from build123d import *

# Parameters (mm, degrees)
MODEL_W                 = 3
MODEL_H                 = 3
SALIENTE_EXTRUIR1_DEPTH = 3


with BuildPart() as part:
    # Model → Saliente-Extruir1 (new body)
    with BuildSketch(Plane.XY):
        with BuildLine():
            Line((12.639309496, 299.028131514), (48.639309496, 299.028131514))
            ThreePointArc((48.639309496, 299.028131514), (51.821290011, 297.71011203), (53.139309496, 294.528131514))
            Line((53.139309496, 294.528131514), (53.139309496, 276.528131514))
            ThreePointArc((53.139309496, 276.528131514), (51.821290011, 273.346150999), (48.639309496, 272.028131514))
            Line((48.639309496, 272.028131514), (12.639309496, 272.028131514))
            ThreePointArc((12.639309496, 272.028131514), (9.457328981, 273.346150999), (8.139309496, 276.528131514))
            Line((8.139309496, 276.528131514), (8.139309496, 294.528131514))
            ThreePointArc((8.139309496, 294.528131514), (9.457328981, 297.71011203), (12.639309496, 299.028131514))
        make_face()
        with Locations((12.639309496, 294.528131514)):
            Rectangle(MODEL_W, MODEL_H, mode=Mode.SUBTRACT)
        with Locations((21.639309496, 294.528131514)):
            Rectangle(MODEL_W, MODEL_H, mode=Mode.SUBTRACT)
        with Locations((30.639309496, 294.528131514)):
            Rectangle(MODEL_W, MODEL_H, mode=Mode.SUBTRACT)
        with Locations((39.639309496, 294.528131514)):
            Rectangle(MODEL_W, MODEL_H, mode=Mode.SUBTRACT)
        with Locations((48.639309496, 294.528131514)):
            Rectangle(MODEL_W, MODEL_H, mode=Mode.SUBTRACT)
        with Locations((12.639309496, 276.528131514)):
            Rectangle(MODEL_W, MODEL_H, mode=Mode.SUBTRACT)
        with Locations((21.639309496, 276.528131514)):
            Rectangle(MODEL_W, MODEL_H, mode=Mode.SUBTRACT)
        with Locations((30.639309496, 276.528131514)):
            Rectangle(MODEL_W, MODEL_H, mode=Mode.SUBTRACT)
        with Locations((39.639309496, 276.528131514)):
            Rectangle(MODEL_W, MODEL_H, mode=Mode.SUBTRACT)
        with Locations((48.639309496, 276.528131514)):
            Rectangle(MODEL_W, MODEL_H, mode=Mode.SUBTRACT)
        with Locations((12.639309496, 285.528131514)):
            Rectangle(MODEL_W, MODEL_H, mode=Mode.SUBTRACT)
        with Locations((21.639309496, 285.528131514)):
            Rectangle(MODEL_W, MODEL_H, mode=Mode.SUBTRACT)
        with Locations((30.639309496, 285.528131514)):
            Rectangle(MODEL_W, MODEL_H, mode=Mode.SUBTRACT)
        with Locations((39.639309496, 285.528131514)):
            Rectangle(MODEL_W, MODEL_H, mode=Mode.SUBTRACT)
        with Locations((48.639309496, 285.528131514)):
            Rectangle(MODEL_W, MODEL_H, mode=Mode.SUBTRACT)
    extrude(amount=SALIENTE_EXTRUIR1_DEPTH)


solid = part.part
Work out the finished part from the listing and answer in its coordinate system (mm). Coordinates: 2 decimals unless noted, no trailing zeros. Order: outer loops, then holes, each group sorted by start corner. A loop starts at its lowest first (then second) coordinate and runs counter-clockwise, first axis right, second up. Notation, with made-up numbers: (61.5, 4.25) - (107.5, 4.25) arc R9 ccw to (107.5, 16.25) - close; hole circle Ø1 at (14, 3.5). An arc over 180 degrees is marked (long way). Put each result on its own line as item: value. Start each with the question number.
1) Find section B-B (z = 2.2). State how many separate pieces and enclosed holes the cut face has, plus the area to 3 significant figures.
2) Find the intervals of material crossed by line 1 (X direction, y = 294, z = 0.45); line 2 (Y direction, x = 30, z = 2.95); line 3 (X direction, y = 295, z = 2.5), in increasing order. Write a range as from..to.
3) Find section A-A (y = 285.75). Give the vertices of the cut face in (x, z).
4) Find section C-C (y = 275.5). Give the vertices of the cut face in (x, z), plus the area to 3 significant figures.
5) For a pull along X with two mould halves and no side action, classify faces 1 (the flat face through (40, 278.028, 1)), 2 (the cylindrical face through (51.79, 297.74, 1.48)) as released by +X, released by -X, zero draft, split by the parting line, or undercut.
Results list:
1. separate pieces: 1
1. enclosed holes: 15
1. area: 1,060 mm^2
2. line 1: x = 8.14..11.14, 14.14..20.14, 23.14..29.14, 32.14..38.14, 41.14..47.14, 50.14..53.14
2. line 2: y = 272.03..275.03, 278.03..284.03, 287.03..293.03, 296.03..299.03
2. line 3: x = 8.16..11.14, 14.14..20.14, 23.14..29.14, 32.14..38.14, 41.14..47.14, 50.14..53.11
3. outline: (8.14, 0) - (11.14, 0) - (11.14, 3) - (8.14, 3) - close; (14.14, 0) - (20.14, 0) - (20.14, 3) - (14.14, 3) - close; (23.14, 0) - (29.14, 0) - (29.14, 3) - (23.14, 3) - close; (32.14, 0) - (38.14, 0) - (38.14, 3) - (32.14, 3) - close; (41.14, 0) - (47.14, 0) - (47.14, 3) - (41.14, 3) - close; (50.14, 0) - (53.14, 0) - (53.14, 3) - (50.14, 3) - close
4. outline: (8.26, 0) - (11.14, 0) - (11.14, 3) - (8.26, 3) - close; (14.14, 0) - (20.14, 0) - (20.14, 3) - (14.14, 3) - close; (23.14, 0) - (29.14, 0) - (29.14, 3) - (23.14, 3) - close; (32.14, 0) - (38.14, 0) - (38.14, 3) - (32.14, 3) - close; (41.14, 0) - (47.14, 0) - (47.14, 3) - (41.14, 3) - close; (50.14, 0) - (53.02, 0) - (53.02, 3) - (50.14, 3) - close
4. area: 89.3 mm^2
5. face 1: undercut
5. face 2: released by +X
